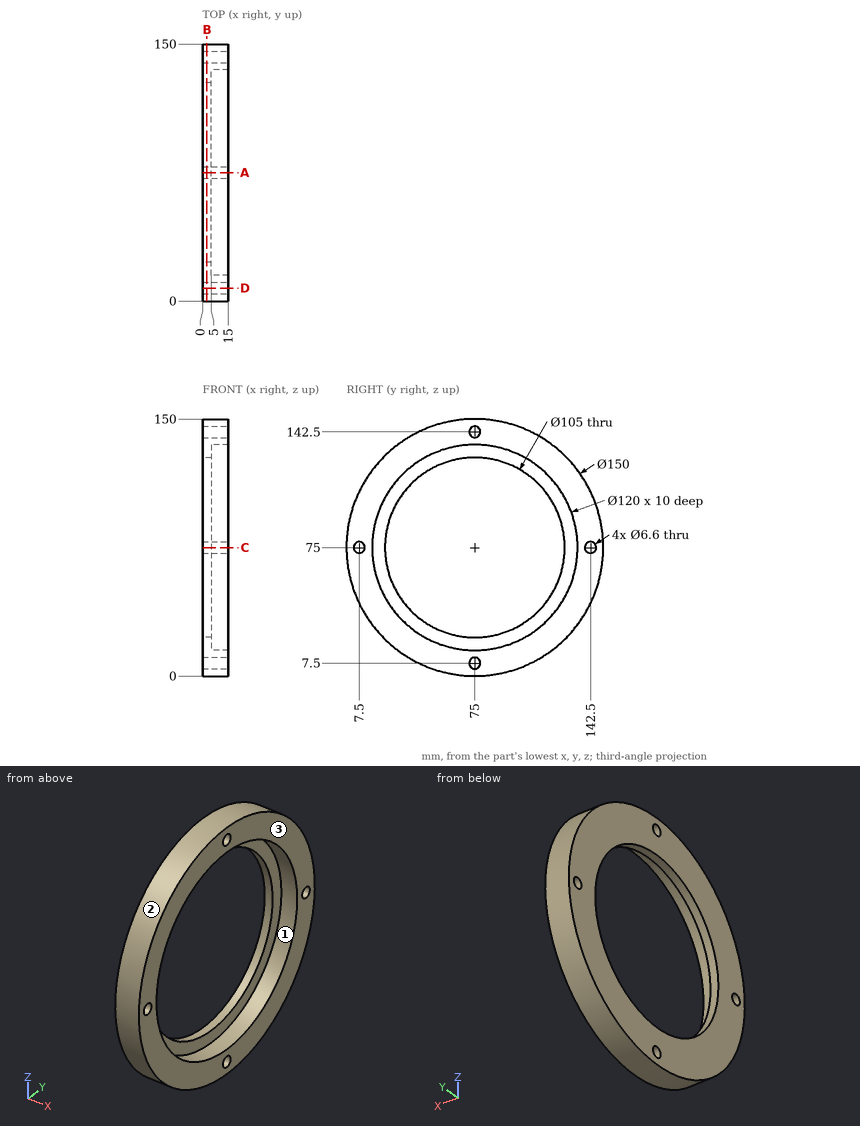
The figure shows three views and two pictorial views of one solid part (mm, origin at its lowest corner). Answer the questions. Round coordinates to 2 decimals unless told otherwise and drop trailing zeros. Write each loop counter-clockwise with the first axis right and the second up, starting at its lowest first coordinate (ties: lowest second). Pieces come first, ordered by that corner, then holes. Notation, with made-up numbers: (14, 54.5) - (55, 54.5) arc R24 ccw to (55, 74.5) - close; hole circle Ø3 at (23, 16.25). An arc over 180 degrees is marked (long way). Answer in a Markdown table with one row per item. Add a question column.
1. Find the intervals of material crossed by line 1 along Y through (x, z) = (1.8, 75); line 2 along Y through (x, z) = (10.25, 75); line 3 along X through (y, z) = (20.5, 57), in increasing order. Write a range as from..to.
2. A cutting plane is placed at A-A, the plane y = 75. Determine the outline of the cut face in (x, z), and give its area (3 significant figures).
3. A cutting plane is placed at D-D, the plane y = 7.5. Determine the outline of the cut face in (x, z).
4. Given pin 1 (4 mm diameter, centred on x = 8, y = 19.5, fed in from +Z); pin 2 (1 mm diameter, centred on x = 12.5, z = 44.5, fed in from +Y); pin 3 (1.5 mm diameter, centred on x = 8.5, y = 134.5, fed in from +Z); pin 4 (5.5 mm diameter, centred on y = 75, z = 142.5, fed in from -X), each flat-ended and moving along its own axis, determine where each tip first touches the part or whether it passes through.
5. A cutting plane is placed at B-B, the plane x = 2.5. Determine the outline of the cut face in (y, z).
6. The mould has two halves that part along Y. Classify the marked faces 1, 2 and 3: +Y half, -Y half, draft (parallel to the pull), parting line (faces both ways), or undercut.
Worked out:
| question | item | result |
|---|---|---|
| 1 | line 1 | 0..4.2, 10.8..22.5, 127.5..139.2, 145.8..150 |
| 1 | line 2 | 0..4.2, 10.8..15, 135..139.2, 145.8..150 |
| 1 | line 3 | 0..5 |
| 2 | outline | (0, 0) - (15, 0) - (15, 4.2) - (0, 4.2) - close; (0, 10.8) - (15, 10.8) - (15, 15) - (5, 15) - (5, 22.5) - (0, 22.5) - close; (0, 127.5) - (5, 127.5) - (5, 135) - (15, 135) - (15, 139.2) - (0, 139.2) - close; (0, 145.8) - (15, 145.8) - (15, 150) - (0, 150) - close |
| 2 | area | 327 mm^2 |
| 3 | outline | (0, 42.31) - (15, 42.31) - (15, 71.7) - (0, 71.7) - close; (0, 78.3) - (15, 78.3) - (15, 107.69) - (0, 107.69) - close |
| 4 | pin 1 | z = 127.56 |
| 4 | pin 2 | y = 143.74 |
| 4 | pin 3 | z = 121.62 |
| 4 | pin 4 | through |
| 5 | outline | circle Ø150 at (75, 75); hole circle Ø6.6 at (7.5, 75); hole circle Ø105 at (75, 75); hole circle Ø6.6 at (75, 7.5); hole circle Ø6.6 at (75, 142.5); hole circle Ø6.6 at (142.5, 75) |
| 6 | face 1 | undercut |
| 6 | face 2 | parting line |
| 6 | face 3 | draft |
